The listing builds one solid part. Answer for the finished solid, in the listing's coordinates (mm). A direction names the side the tool comes from. Round coordinates to 2 decimals unless told otherwise and drop trailing zeros. Loops run counter-clockwise (first coordinate to the right, second up) from the corner with the lowest first, then second, coordinate; pieces in that order, holes last. Notation, with made-up numbers: (48.5, 12) -> (82.5, 12) arc R20 ccw to (82.5, 27) -> close; hole circle Ø10 at (52, 86). An arc over 180 degrees is marked (long way). One line per question, with ' | ' between items.
from build123d import *

# Parameters (mm, degrees)
F0_W      = 482.6
F0_H      = 482.6
F1_DEPTH  = 12.8524
F2_W      = 330.2
F2_H      = 12.8524
F2_W_2    = 76.2
F3_DEPTH  = 50.8
F4_W      = 330.2
F4_H      = 12.8524
F4_W_2    = 76.2
F5_DEPTH  = 50.8
F8_W      = 127
F8_H      = 74.67717
F8_H_2    = 75.18283
F9_W      = 127
F9_H      = 74.67717
F10_DEPTH = 25.4
F12_R     = 13.2461
F12_R_2   = 30.353
F13_DEPTH = 25.4


with BuildPart() as f1:
    # F0 (on Top) → F1 (new body)
    with BuildSketch(Plane.XY):
        with Locations((-241.3, -241.3)):
            Rectangle(F0_W, F0_H)
    extrude(amount=F1_DEPTH)

    # F2 (on face) → F3 (cut)
    with BuildSketch(Plane.XZ.offset(482.6)):
        with Locations((-241.3, 6.4262)):
            Rectangle(F2_W, F2_H)
        with Locations((-444.5, 6.4262)):
            Rectangle(F2_W_2, F2_H)
    extrude(amount=-F3_DEPTH, mode=Mode.SUBTRACT)

    # F4 (on face) → F5 (cut)
    with BuildSketch(Plane(origin=(0, 0, 0), x_dir=(-1, 0, 0), z_dir=(0, 1, 0))):
        with Locations((241.3, 6.4262)):
            Rectangle(F4_W, F4_H)
        with Locations((38.1, 6.4262)):
            Rectangle(F4_W_2, F4_H)
    extrude(amount=-F5_DEPTH, mode=Mode.SUBTRACT)

    # F8 (on face) + F9 (on face) → F10 (cut)
    with BuildSketch(Plane.XY.offset(12.8524)):
        with Locations((-139.7, -318.261415)):
            Rectangle(F8_W, F8_H)
        with Locations((-342.9, -164.591415)):
            Rectangle(F8_W, F8_H_2)
        with Locations((-139.7, -164.591415)):
            Rectangle(F8_W, F8_H_2)
    with BuildSketch(Plane.XY.offset(12.8524)):
        with Locations((-342.9, -318.261415)):
            Rectangle(F9_W, F9_H)
    extrude(amount=-F10_DEPTH, mode=Mode.SUBTRACT)

    # F12 (on face) → F13 (cut)
    with BuildSketch(Plane.XY.offset(12.8524)):
        with Locations((-444.285613, -28.4861)):
            Circle(F12_R)
        with Locations((-241.3, -241.55283)):
            Circle(F12_R_2)
        with Locations((-38.0111, -454.1139)):
            Circle(F12_R)
    extrude(amount=-F13_DEPTH, mode=Mode.SUBTRACT)


solid = f1.part
Q1. For a pull along Y with two mould halves and no side action, classify faces 1 (the face through (-406.4, -25, 6)), 2 (the face through (-445, 0, 6)), 3 (the face through (-279.4, -319, 7)) as pulls with the +Y half, pulls with the -Y half, needs draft (parallel to the pull), parting line crosses it, or undercut.
Numbers:
face 1: needs draft | face 2: pulls with the +Y half | face 3: undercut
Q2. A cutting plane is placed at B-B on x = -103.5. Give the vertices of the cut face in (y, z), plus the area to 3 significant figures.
Numbers:
outline: (-431.8, 0) -> (-355.6, 0) -> (-355.6, 12.85) -> (-431.8, 12.85) -> close; (-280.92, 0) -> (-202.18, 0) -> (-202.18, 12.85) -> (-280.92, 12.85) -> close; (-127, 0) -> (-50.8, 0) -> (-50.8, 12.85) -> (-127, 12.85) -> close | area: 2,970 mm^2
Q3. A cutting plane is placed at A-A on x = -241.3. Give the vertices of the cut face in (y, z), plus the area to 3 significant figures.
Numbers:
outline: (-431.8, 0) -> (-271.91, 0) -> (-271.91, 12.85) -> (-431.8, 12.85) -> close; (-211.2, 0) -> (-50.8, 0) -> (-50.8, 12.85) -> (-211.2, 12.85) -> close | area: 4,120 mm^2
Q4. For faces 4 (the face through (-344, -280.923, 7)), 5 (the face through (-282, -431.8, 7)), 6 (the face through (-482.6, -219, 6)), determine the directions among +Z, -Z, +X, -X, +Y, -Y from which every point of the face is accessible in a straight line to the end or side of a thin tool.
Numbers:
face 4: +Z, -Z | face 5: +Z, -Z, -X, -Y | face 6: +Z, -Z, -X, +Y, -Y
Q5. A cutting plane is placed at C-C on z = 4. Give the vertices of the cut face in (x, y) (3 decimals).
Numbers:
outline: (-482.6, -431.8) -> (-76.2, -431.8) -> (-76.2, -482.6) -> (0, -482.6) -> (0, -50.8) -> (-406.4, -50.8) -> (-406.4, 0) -> (-482.6, 0) -> close; hole circle Ø26.492 at (-444.286, -28.486); hole (-406.4, -355.6) -> (-279.4, -355.6) -> (-279.4, -280.923) -> (-406.4, -280.923) -> close; hole (-406.4, -202.183) -> (-279.4, -202.183) -> (-279.4, -127) -> (-406.4, -127) -> close; hole circle Ø60.706 at (-241.3, -241.553); hole (-203.2, -355.6) -> (-76.2, -355.6) -> (-76.2, -280.923) -> (-203.2, -280.923) -> close; hole (-203.2, -202.183) -> (-76.2, -202.183) -> (-76.2, -127) -> (-203.2, -127) -> close; hole circle Ø26.492 at (-38.011, -454.114)
Q6. Given pin 1 Ø6.5 at (y, z) = (-454, 8.5) entering from -X; pin 2 Ø1.5 at (x, z) = (-384.5, 7) entering from -Y; pin 3 Ø8 at (x, y) = (-174.5, -240) entering from -Z; pin 4 Ø6.5 at (x, z) = (-114, 8) entering from +Y, each flat-ended and moving along its own axis, determine where each tip first touches the part or whether it passes through.
Numbers:
pin 1: x = -76.2 | pin 2: y = -431.8 | pin 3: z = 0 | pin 4: y = -50.8
Q7. Find the intervals of material crossed by line 1 (Y direction, x = -196, z = 2.25); line 2 (X direction, y = -316, z = 11.25); line 3 (X direction, y = -34, z = 9.5), in increasing order. Write a range as from..to.
Numbers:
line 1: -431.8..-355.6, -280.92..-202.18, -127..-50.8 | line 2: -482.6..-406.4, -279.4..-203.2, -76.2..0 | line 3: -482.6..-456.33, -432.24..-406.4
